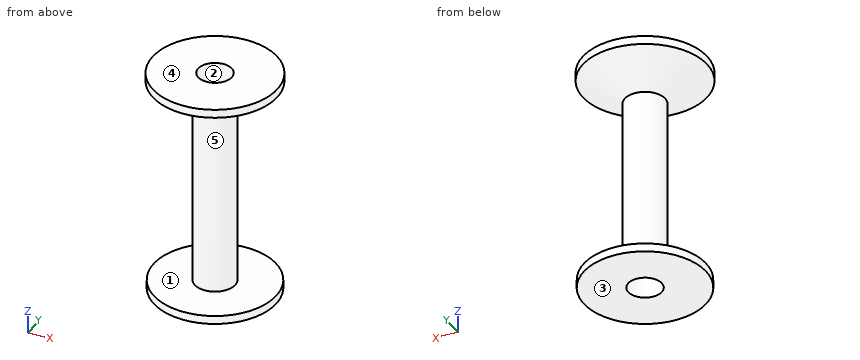
```python
from build123d import *

# Parameters (mm, degrees)
F2_SIZE2 = 5.773493
F2_SIZE  = 9.99999


# Not quite as in the source:
# - a fillet or chamfer is up to 0.001 mm smaller than in the source, because OpenCascade refuses the exact size


with BuildPart() as f1:
    # F0 (on Front) → F1 (revolve)
    with BuildSketch(Plane.XZ):
        Polygon((-14.5480483851, 0), (-4, 0), (-4, 54), (-14.8, 54), (-14.8, 52), (-4.8, 52), (-4.8, 2), (-14.5480483851, 2), align=None)
    revolve(axis=Axis((0, 0, 27), (0, 0, -1)))

    # F2 (size 10 and 5.7735026919 in the source; OpenCascade refuses exactly that, so slightly less here)
    f2_edges = [f1.edges().sort_by_distance(p)[0] for p in [
        (4.8, 0, 52),
    ]]
    chamfer(f2_edges, length=F2_SIZE, length2=F2_SIZE2)


solid = f1.part
```
The listing builds one solid part. Answer for the finished solid, in the listing's coordinates (mm). Face numbers are marked on the shaded views. A direction names the side the tool comes from. Give positions to 0.01 mm unless a question says otherwise; leave off trailing zeros. Loops run counter-clockwise (first coordinate to the right, second up) from the corner with the lowest first, then second, coordinate; pieces in that order, holes last. Notation, with made-up numbers: M 82,22.25 L 116,22.25 A17 cw 116,33.25 Z; hole C 75,28 d5. An arc over 180 degrees is marked long. One line per item, written item: value.
1. For a pull along Z with two mould halves and no side action, classify the marked faces 1, 2 and 3 as pulls with the +Z half, pulls with the -Z half, needs draft (parallel to the pull), parting line crosses it, or undercut.
Found:
face 1: undercut
face 2: needs draft
face 3: pulls with the -Z half
2. Section C-C on z = 19.5 is taken. Determine the outline of the cut face in (x, y).
Found:
outline: C 0,0 d9.6; hole C 0,0 d8
3. Each of these flat-tipped pins is pushed along its axis until it touches: P1, Ø2, axis at x = 7.5, z = 33.5, coming from the -Y side; P2, Ø1.5, axis at x = 3.5, z = 18, coming from the -Y side; P3, Ø3, axis at y = -1.5, z = 23, coming from the +X side. Where does it stop, or does it pass through?
Found:
P1: through
P2: y = -3.93
P3: x = 4.8
4. For the marked faces 4 and 5, determine the directions among +Z, -Z, +X, -X, +Y, -Y from which every point of the face is accessible in a straight line to the end or side of a thin tool.
Found:
face 4: +Z, +X, -X, +Y, -Y
face 5: none
5. Find the intervals of material crossed by probe 1 along Y at (x, z) = (0, 18.5); probe 2 along Z at (x, y) = (12.75, -6); probe 3 along X at (y, z) = (-3.25, 43), in increasing order.
Found:
probe 1: -4.8 to -4, 4 to 4.8
probe 2: 0 to 2, 51.59 to 54
probe 3: -3.53 to -2.33, 2.33 to 3.53
